```python
from build123d import *

# Parameters (mm, degrees)
SKETCH2_R          = 6.5
SKETCH2_R_2        = 7.75
CUT_EXTRUDE1_DEPTH = 119.521470637


with BuildPart() as part:
    # Sketch1 → Revolve1 (revolve)
    with BuildSketch(Plane(origin=(0, 0, 0), x_dir=(0, 0, -1), z_dir=(1, 0, 0)), mode=Mode.PRIVATE) as revolve1_sk:
        with BuildLine():
            Line((0, 0), (0, 76.444627725))
            ThreePointArc((0, 76.444627725), (0.130798304, 76.879222907), (0.479738309, 77.169433247))
            Line((0.479738309, 77.169433247), (0.872854821, 77.336301306))
            ThreePointArc((0.872854821, 77.336301306), (1.6002, 78.4352), (0.872854821, 79.534098694))
            Line((0.872854821, 79.534098694), (0.479738309, 79.700966753))
            ThreePointArc((0.479738309, 79.700966753), (0.130798304, 79.991177093), (0, 80.425772275))
            Line((0, 80.425772275), (0, 83.439))
            Line((0, 83.439), (5.588, 83.439))
            Line((5.588, 83.439), (11.0998, 68.295453959))
            Line((11.0998, 68.295453959), (11.0998, 0))
            Line((11.0998, 0), (0, 0))
        make_face()
    revolve(revolve1_sk.sketch.rotate(Axis((0, 0, 0), (0, 0, -1)), 90), axis=Axis((0, 0, 0), (0, 0, -1)))

    # Sketch2 → Cut-Extrude1 (cut, through all)
    with BuildSketch(Plane(origin=(0, 0, -11.0998), x_dir=(-1, 0, 0), z_dir=(0, 0, -1))):
        Circle(SKETCH2_R)
        with Locations((0, 27.9765569)):
            Circle(SKETCH2_R_2)
        with Locations((-24.324092368, 0)):
            Circle(SKETCH2_R)
        with Locations((24.098999837, -10.15759269)):
            Circle(SKETCH2_R)
        with Locations((-24.324092368, 24.067370628)):
            Circle(SKETCH2_R)
        with Locations((21.259374059, 15.100131331)):
            Circle(SKETCH2_R)
        with Locations((-4.297257938, -26.149169437)):
            Circle(SKETCH2_R_2)
        with Locations((-28.209896064, -23.907359612)):
            Circle(SKETCH2_R)
        with Locations((18.120840305, -33.771322839)):
            Circle(SKETCH2_R_2)
    extrude(amount=-CUT_EXTRUDE1_DEPTH, mode=Mode.SUBTRACT)


solid = part.part
```
Design review of the part built by this model. Coordinates are the model's own, in mm. Give positions to 0.01 mm unless a question says otherwise; leave off trailing zeros. Loops run counter-clockwise (first coordinate to the right, second up) from the corner with the lowest first, then second, coordinate; pieces in that order, holes last. Notation, with made-up numbers: (35.25, 19.25) -> (44.25, 19.25) arc R18 ccw to (44.25, 54.25) -> close; hole circle Ø1 at (-34.5, 25). An arc over 180 degrees is marked (long way). Write each question's results on one line, items separated by ' | '.
Q1. Take a section at B-B, the plane x = 0. Give the number of separate pieces and of enclosed holes in the cut face, plus the area to 3 significant figures.
Reply:
separate pieces: 4 | enclosed holes: 0 | area: 1,300 mm²
Q2. For pin 1 Ø2 at (x, z) = (-27, -3) entering from -Y; pin 2 Ø4 at (y, z) = (-63.5, -2.5) entering from -X; pin 3 Ø5 at (y, z) = (19.5, -4.5) entering from -X, all flat-tipped, find the tip position at first contact; note any pin that passes through.
Reply:
pin 1: stops at y = -79.28 | pin 2: stops at x = -56.39 | pin 3: stops at x = -81.69
Q3. Take a section at A-A, the plane y = 0. Write out the cut boundary in (x, z), plus the area to 3 significant figures.
Reply:
outline: (-83.44, -5.59) -> (-68.3, -11.1) -> (-6.5, -11.1) -> (-6.5, 0) -> (-76.44, 0) arc R0.79 ccw to (-77.17, -0.48) -> (-77.34, -0.87) arc R1.19 cw to (-79.53, -0.87) -> (-79.7, -0.48) arc R0.79 ccw to (-80.43, 0) -> (-83.44, 0) -> close; (6.5, -11.1) -> (17.82, -11.1) -> (17.82, 0) -> (6.5, 0) -> close; (30.82, -11.1) -> (68.3, -11.1) -> (83.44, -5.59) -> (83.44, 0) -> (80.43, 0) arc R0.79 ccw to (79.7, -0.48) -> (79.53, -0.87) arc R1.19 cw to (77.34, -0.87) -> (77.17, -0.48) arc R0.79 ccw to (76.44, 0) -> (30.82, 0) -> close | area: 1,470 mm²
Q4. The part is to be moulded in two halves that separate along X. For faces 1 (the face through (1, 16, 0)), 2 (the face through (-8.986, -68.443, -10.832)), 3 (the face through (34.704, -23.622, -5.628)), 4 (the face through (-24.754, 20.581, -5.628)), say which applies: +X half, -X half, draft (parallel to the pull), parting line (faces both ways), or undercut.
Reply:
face 1: draft | face 2: parting line | face 3: undercut | face 4: undercut
Q5. Wall thickness on L1, parallel to Y at x = 36, z = -1; L2, parallel to X at y = -51.5, z = -0.25; L3, parallel to X at y = 15, z = -0.75: over which ranges is each line inside the solid? List them lowest first.
Reply:
L1: y = -75.27 to -70.85, -68.52 to 68.52, 70.85 to 75.27 | L2: x = -65.65 to -61.02, -57.27 to 57.27, 61.02 to 65.65 | L3: x = -82.08 to -78.16, -75.81 to -27.76, -14.76 to 75.81, 78.16 to 82.08
